Geometry check sheet. Reference: the model listing, model coordinates, mm. A direction names the side the tool comes from. Round coordinates to 2 decimals unless told otherwise and drop trailing zeros. Write each loop counter-clockwise with the first axis right and the second up, starting at its lowest first coordinate (ties: lowest second). Pieces come first, ordered by that corner, then holes. Notation, with made-up numbers: (16, 59.5) -> (45, 59.5) arc R10 cw to (45, 64.5) -> close; hole circle Ø2 at (-11.75, -31.75). An arc over 180 degrees is marked (long way). Use a Markdown table: item, result.
```python
from build123d import *

# Parameters (mm, degrees)
PAD_DEPTH           = 30
SKETCH001_R         = 6
POCKET_DEPTH        = 11
SKETCH002_R         = 2
POCKET001_DEPTH     = 5
LINEARPATTERN_COUNT = 2
LINEARPATTERN_PITCH = 28
PAD001_DEPTH        = 30


with BuildPart() as part:
    # Sketch → Pad (new body)
    with BuildSketch(Plane.XY):
        with BuildLine():
            Line((0, 20), (-84, 20))
            ThreePointArc((-84, 20), (-104, 0), (-84, -20))
            Line((0, -20), (-84, -20))
            Line((0, 20), (0, -20))
        make_face()
    extrude(amount=PAD_DEPTH)

    # Sketch001 (on Face6 of Pad) → Pocket (cut)
    with BuildSketch(Plane.XY.offset(30)):
        with Locations((-84, 0)):
            Circle(SKETCH001_R)
    extrude(amount=-POCKET_DEPTH, mode=Mode.SUBTRACT)

    # Sketch002 (on Face5 of Pocket) → Pocket001 (cut)
    with BuildSketch(Plane.XY.offset(30)):
        with Locations((-56, 0)):
            Circle(SKETCH002_R)
    pocket001 = extrude(amount=-POCKET001_DEPTH, mode=Mode.SUBTRACT)

    # LinearPattern: Pocket001 ×2
    with Locations(*[(i * LINEARPATTERN_PITCH, 0, 0) for i in range(1, LINEARPATTERN_COUNT)]):
        add(pocket001, mode=Mode.SUBTRACT)

    # Sketch003 (on Face5 of LinearPattern) → Pad001 (join)
    with BuildSketch(Plane.XY.offset(30)):
        with BuildLine():
            Line((-30.44, -14.81438), (-30.44, 0))
            ThreePointArc((-30.44, 0), (-18.638963, 3.884356), (-13.414303, 15.156251))
            Line((0, 20), (-13.414303, 15.156251))
            Line((0, -20), (0, 20))
            Line((-30.44, -14.81438), (0, -20))
        make_face()
    extrude(amount=PAD001_DEPTH)


solid = part.part
```
(1) Section check A-A on z = 27.5. Record the cut outline in (x, y), plus the area to 3 significant figures.
A:
| item | result |
|---|---|
| outline | (-84, -20) -> (0, -20) -> (0, 20) -> (-84, 20) arc R20 ccw to start; hole circle Ø12 at (-84, 0); hole circle Ø4 at (-56, 0); hole circle Ø4 at (-28, 0) |
| area | 3,850 mm2 |
(2) Gauge pin test, flat ends, axial feed: pin 1 Ø8 at (x, y) = (-22.5, 14.5) entering from +Z; pin 2 Ø3.5 at (x, y) = (-84.5, -2.5) entering from +Z; pin 3 Ø16.5 at (y, z) = (-4.5, 48.5) entering from -X. Record the tip position at first contact, or that the pin passes through.
A:
| item | result |
|---|---|
| pin 1 | stops at z = 30 |
| pin 2 | stops at z = 19 |
| pin 3 | stops at x = -30.44 |
(3) Release check for a two-part mould opening along Y. For faces 4 (the face through (-6.613, 17.612, 44.79)), 5 (the face through (-26.153, -0.766, 27.535)), 6 (the face through (-104, 0, 15)), 7 (the face through (-12, -4, 60)) record: +Y half, -Y half, draft (parallel to the pull), parting line (faces both ways), or undercut.
A:
| item | result |
|---|---|
| face 4 | +Y half |
| face 5 | undercut |
| face 6 | parting line |
| face 7 | draft |
(4) Section check B-B on x = -56. Record the cut outline in (y, z).
A:
| item | result |
|---|---|
| outline | (-20, 0) -> (20, 0) -> (20, 30) -> (2, 30) -> (2, 25) -> (-2, 25) -> (-2, 30) -> (-20, 30) -> close |
(5) Section check C-C on y = -10.5. Record the cut outline in (x, z), plus the area to 3 significant figures.
A:
| item | result |
|---|---|
| outline | (-101.02, 0) -> (0, 0) -> (0, 60) -> (-30.44, 60) -> (-30.44, 30) -> (-101.02, 30) -> close |
| area | 3,940 mm2 |
(6) Section check D-D on x = -28. Record the cut outline in (y, z), plus the area to 3 significant figures.
A:
| item | result |
|---|---|
| outline | (-20, 0) -> (20, 0) -> (20, 30) -> (2, 30) -> (2, 25) -> (-2, 25) -> (-2, 30) -> (-0.03, 30) -> (-0.03, 60) -> (-15.23, 60) -> (-15.23, 30) -> (-20, 30) -> close |
| area | 1,640 mm2 |
(7) Access from +Z, -Z, +X, -X, +Y, -Y to the whole of each face (thin tool, end or side, straight path). Record for faces 1 (the face through (-15.43, -17.37, 44.79)), 2 (the face through (-58, 0, 28)), 3 (the face through (-28, -1, 30)).
A:
| item | result |
|---|---|
| face 1 | +Z, -X, -Y |
| face 2 | +Z |
| face 3 | none |
(8) Thickness scan on line 1 (Y direction, x = -56, z = 27.2); line 2 (Z direction, x = -20, y = 17); line 3 (Y direction, x = -84, z = 22.75). Record the ranges inside material, lowest first.
A:
| item | result |
|---|---|
| line 1 | y = -20 to -2, 2 to 20 |
| line 2 | z = 0 to 30 |
| line 3 | y = -20 to -6, 6 to 20 |
